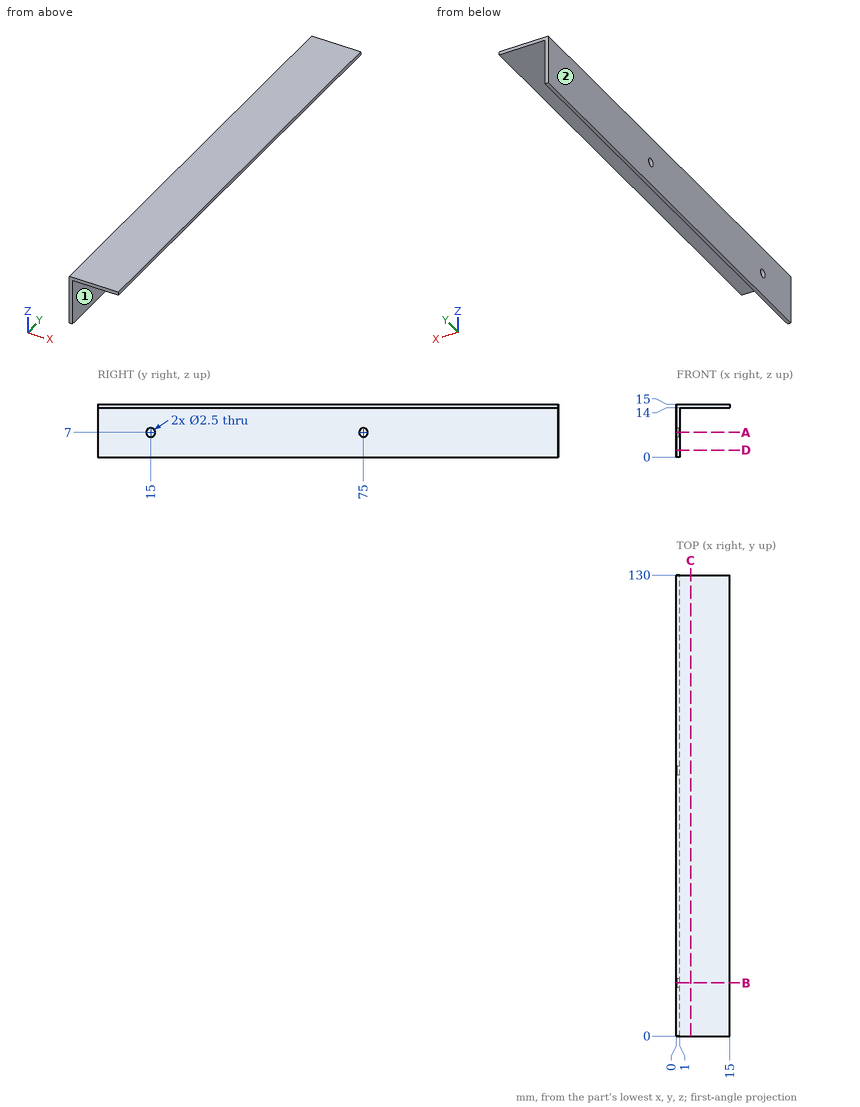
Study the drawing (mm; zero at the part's minimum x, y, z) and answer. A direction names the side the tool comes from. Give positions to 0.01 mm unless a question says otherwise; leave off trailing zeros. Order: outer loops, then holes, each group sorted by start corner. A loop starts at its lowest first (then second) coordinate and runs counter-clockwise, first axis right, second up. Notation, with made-up numbers: (-23.5, 60) - (29.5, 60) arc R22 ccw to (29.5, 84) - close; hole circle Ø2 at (3.25, 47). An arc over 180 degrees is marked (long way). Answer as CSV lines item,"result". Start each with the question number.
Q1. Find the intervals of material crossed by L1, parallel to Y at x = 0.85, z = 7; L2, parallel to Z at x = 0.7, y = 75; L3, parallel to Z at x = 5, y = 103.5, in increasing order. Write a range as [from, to].
Q2. The part is cut by section D-D (z = 2). Write down the section's boundary in (x, y), then the cut area to 3 significant figures.
Q3. The part is cut by section B-B (y = 15). Write down the section's boundary in (x, z), then the cut area to 3 significant figures.
Q4. For the marked faces 1 and 2, determine the directions among +Z, -Z, +X, -X, +Y, -Y from which every point of the face is accessible in a straight line to the end or side of a thin tool.
Q5. Given pin 1 Ø3 at (y, z) = (77.5, 2) entering from -X; pin 2 Ø4 at (x, y) = (8.5, 45.5) entering from -Z; pin 3 Ø3 at (y, z) = (75, 7) entering from +X, each flat-ended and moving along its own axis, determine where each tip first touches the part or whether it passes through.
Q6. The part is cut by section A-A (z = 7). Write down the section's boundary in (x, y), then the cut area to 3 significant figures.
Q7. The part is cut by section C-C (x = 4). Write down the section's boundary in (y, z), then the cut area to 3 significant figures.
Check result:
1,L1,"y = [0, 13.75], [16.25, 73.75], [76.25, 130]"
1,L2,"z = [0, 5.75], [8.25, 15]"
1,L3,"z = [14, 15]"
2,outline,"(0, 0) - (1, 0) - (1, 130) - (0, 130) - close"
2,area,"130 mm²"
3,outline,"(0, 0) - (1, 0) - (1, 5.75) - (0, 5.75) - close; (0, 8.25) - (1, 8.25) - (1, 14) - (15, 14) - (15, 15) - (0, 15) - close"
3,area,"26.5 mm²"
4,face 1,"-Z, +X, +Y, -Y"
4,face 2,"+Z, -Z, -X, +Y, -Y"
5,pin 1,"stops at x = 0"
5,pin 2,"stops at z = 14"
5,pin 3,"stops at x = 1"
6,outline,"(0, 0) - (1, 0) - (1, 13.75) - (0, 13.75) - close; (0, 16.25) - (1, 16.25) - (1, 73.75) - (0, 73.75) - close; (0, 76.25) - (1, 76.25) - (1, 130) - (0, 130) - close"
6,area,"125 mm²"
7,outline,"(0, 14) - (130, 14) - (130, 15) - (0, 15) - close"
7,area,"130 mm²"
